from build123d import *

# Parameters (mm, degrees)
F0_W = 11.223247965
F0_H = 25.4
F2_T = -2.54
F4_R = 5.08


# Not quite as in the source:
# - a fillet or chamfer that OpenCascade refuses, or shapes differently, is made with other operations: its cross-section is extruded or revolved along the edge and cut away or added


with BuildPart() as f1:
    # F0 (on Top) → F1 (revolve)
    with BuildSketch(Plane.XY):
        with Locations((5.6116239825, 12.7)):
            Rectangle(F0_W, F0_H)
    revolve(axis=Axis((0, 12.7, 0), (0, 1, 0)))

    # F2
    f2_openings = [f1.faces().sort_by_distance(p)[0] for p in [
        (0, 25.4, 0),
    ]]
    offset(amount=F2_T, openings=f2_openings)

    # F3: fillet of radius 5.08 on 1 edges, made by hand

    # F3_s1 → F3_t2 (revolve, cut)
    with BuildSketch(Plane.XY):
        with BuildLine():
            ThreePointArc((11.223247965, 25.4), (9.3638389137, 23.5405909488), (8.683247965, 21.0005909488))
            Line((8.683247965, 21.0005909488), (8.581647965, 21.0005909488))
            Line((8.581647965, 21.0005909488), (8.581647965, 25.4))
            Line((8.581647965, 25.4), (8.683247965, 25.5016))
            ThreePointArc((8.683247965, 25.5016), (9.953247965, 25.5016), (11.172447965, 25.487988181))
            Line((11.172447965, 25.487988181), (11.223247965, 25.4))
        make_face()
    revolve(axis=Axis((0, 25.4, 0), (0, 1, 0)), mode=Mode.SUBTRACT)

    # F4
    f4_edges = [f1.edges().sort_by_distance(p)[0] for p in [
        (-11.223248, 0, 0),
    ]]
    fillet(f4_edges, radius=F4_R)


solid = f1.part
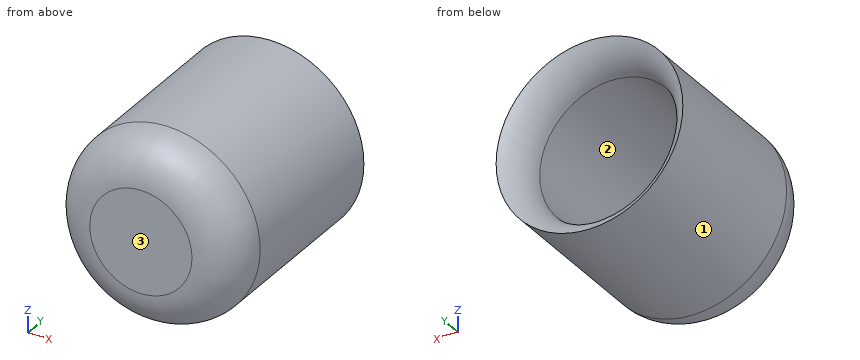
For this review, take the finished solid that the model builds, in its own axes (mm). Face numbers are marked on the shaded views. Coordinates: 2 decimals unless noted, no trailing zeros. Write each loop counter-clockwise with the first axis right and the second up, starting at its lowest first coordinate (ties: lowest second). Pieces come first, ordered by that corner, then holes. Notation, with made-up numbers: (82.25, 38) -> (97.25, 38) arc R11 ccw to (97.25, 53) -> close; hole circle Ø10 at (83.5, -17.5). An arc over 180 degrees is marked (long way). Write each question's results on one line, items separated by ' | '. Start each with the question number.
1) Insertion check: pin 1 (12 mm diameter, centred on x = 7.5, y = 8, fed in from +Z); pin 2 (6 mm diameter, centred on x = 8, y = 22, fed in from +Z); pin 3 (1.5 mm diameter, centred on x = 7, y = 21, fed in from +Z). Each pin has a flat end and moves straight along its axis. Give the tip position at first contact, or say it passes through.
2) The part is to be moulded in two halves that separate along X. For the marked faces 1, 2 and 3, say which applies: +X half, -X half, draft (parallel to the pull), parting line (faces both ways), or undercut.
3) Wall thickness on L1, parallel to X at y = 15, z = 0; L2, parallel to Z at x = 7.5, y = 22.5: over which ranges is each line inside the solid? List them lowest first. Write a range as [from, to].
4) Consider section B-B (z = 0). Write out the cut boundary in (x, y).
5) Consider section C-C (y = 5.5). Write out the cut boundary in (x, z).
6) Consider section A-A (x = 0). Write out the cut boundary in (y, z), plus the area to 3 significant figures.
7) Consider section D-D (y = 1.75). Write out the cut boundary in (x, z).
Geometry says:
1) pin 1: z = 11.12 | pin 2: z = 10.05 | pin 3: z = 9.32
2) face 1: parting line | face 2: undercut | face 3: draft
3) L1: [-11.22, -8.68], [8.68, 11.22] | L2: [-8.35, -4.81], [4.81, 8.35]
4) outline: (-11.22, 5.08) arc R5.08 ccw to (-6.14, 0) -> (6.14, 0) arc R5.08 ccw to (11.22, 5.08) -> (11.22, 25.4) arc R5.08 ccw to (8.68, 21) -> (8.68, 2.54) -> (-8.68, 2.54) -> (-8.68, 21) arc R5.08 ccw to (-11.22, 25.4) -> close
5) outline: circle Ø22.45 at (0, 0); hole circle Ø17.37 at (0, 0)
6) outline: (0, -6.14) arc R5.08 ccw to (5.08, -11.22) -> (25.4, -11.22) arc R5.08 ccw to (21, -8.68) -> (2.54, -8.68) -> (2.54, 8.68) -> (21, 8.68) arc R5.08 ccw to (25.4, 11.22) -> (5.08, 11.22) arc R5.08 ccw to (0, 6.14) -> close | area: 156 mm^2
7) outline: circle Ø19.96 at (0, 0)
